Work out the finished part from the listing and answer in its coordinate system (mm). A direction names the side the tool comes from. Give positions to 0.01 mm unless a question says otherwise; leave off trailing zeros. Write each loop counter-clockwise with the first axis right and the second up, starting at its lowest first coordinate (ties: lowest second). Pieces come first, ordered by that corner, then holes.
1) Find section B-B (y = 9). Determine the outline of the cut face in (x, z).
2) Straight lines are drawn through the part: probe 1 along Y at (x, z) = (8.5, 5); probe 2 along X at (y, z) = (2.5, 2.5); probe 3 along Y at (x, z) = (51, 9.25). For each, find the intervals that lie inside material, in ascending order.
3) Given pin 1 Ø9.5 at (x, y) = (10.5, 6.5) entering from +Z; pin 2 Ø1 at (x, y) = (45, -1) entering from +Z; pin 3 Ø1.2 at (y, z) = (2.5, 5) entering from +X, each flat-ended and moving along its own axis, determine where each tip first touches the part or whether it passes through.
4) Find section C-C (z = 1.75). Determine the outline of the cut face in (x, y).
5) Find section D-D (z = 12.5). Determine the outline of the cut face in (x, y).
6) A tool of negligible diameter and unlimited length cuts with its end or side. For faces 4 (the face through (53.5, 6, 5)), 5 (the face through (65, 9, 5)), 6 (the face through (38, 0, 12)), from which of +Z, -Z, +X, -X, +Y, -Y can it reach the whole face along a straight path? Write none if from no direction.
7) Find section A-A (x = 49). Determine the outline of the cut face in (y, z), plus the area to 3 significant figures.
8) Determine the mould class of faces 1 (the face through (38, -5, 10)), 2 (the face through (65, -2, 20)), 3 (the face through (12, 3, 5)) for opening direction Y: pulls with the +Y half, pulls with the -Y half, needs draft (parallel to the pull), parting line crosses it, or undercut.
```python
from build123d import *

# Parameters (mm, degrees)
SKETCH1_W           = 77
SKETCH1_H           = 12
BOSS_EXTRUDE1_DEPTH = 10
SKETCH2_R           = 1.25
CUT_EXTRUDE1_DEPTH  = 12
SKETCH3_W           = 77
SKETCH3_H           = 20
BOSS_EXTRUDE2_DEPTH = 5
SKETCH4_W           = 30
SKETCH4_H           = 6
CUT_EXTRUDE2_DEPTH  = 10
SKETCH5_W           = 30
SKETCH5_H           = 2.5
CUT_EXTRUDE3_DEPTH  = 5


with BuildPart() as part:
    # Sketch1 → Boss-Extrude1 (new body)
    with BuildSketch(Plane.XY):
        with Locations((38.5, 6)):
            Rectangle(SKETCH1_W, SKETCH1_H)
    extrude(amount=BOSS_EXTRUDE1_DEPTH)

    # Sketch2 → Cut-Extrude1 (cut)
    with BuildSketch(Plane(origin=(77, 0, 0), x_dir=(0, 0, -1), z_dir=(1, 0, 0))):
        with Locations((-5, 3)):
            Circle(SKETCH2_R)
        with Locations((-5, 9)):
            Circle(SKETCH2_R)
    cut_extrude1 = extrude(amount=-CUT_EXTRUDE1_DEPTH, mode=Mode.SUBTRACT)

    # Mirror1: Cut-Extrude1 across plane
    add(cut_extrude1.mirror(Plane.ZY.offset(-38.5)), mode=Mode.SUBTRACT)

    # Sketch3 → Boss-Extrude2 (add)
    with BuildSketch(Plane(origin=(0, 12, 0), x_dir=(1, 0, 0), z_dir=(0, 1, 0))):
        with Locations((38.5, -10)):
            Rectangle(SKETCH3_W, SKETCH3_H)
    boss_extrude2 = extrude(amount=BOSS_EXTRUDE2_DEPTH)

    # Mirror2: Boss-Extrude2 across plane
    add(boss_extrude2.mirror(Plane(origin=(0, 6, 0), x_dir=(0, 0, 1), z_dir=(0, -1, 0))))

    # Sketch4 → Cut-Extrude2 (cut)
    with BuildSketch(Plane(origin=(0, 0, 0), x_dir=(-1, 0, 0), z_dir=(0, 0, -1))):
        with Locations((-38.5, 9)):
            Rectangle(SKETCH4_W, SKETCH4_H)
        with Locations((-38.5, 3)):
            Rectangle(SKETCH4_W, SKETCH4_H)
    extrude(amount=-CUT_EXTRUDE2_DEPTH, mode=Mode.SUBTRACT)

    # Sketch5 → Cut-Extrude3 (cut)
    with BuildSketch(Plane.XY.offset(20)):
        with Locations((38.5, -1.25)):
            Rectangle(SKETCH5_W, SKETCH5_H)
        with Locations((38.5, -3.75)):
            Rectangle(SKETCH5_W, SKETCH5_H)
    extrude(amount=-CUT_EXTRUDE3_DEPTH, mode=Mode.SUBTRACT)


solid = part.part
```
Results:
1. outline: (0, 0) - (23.5, 0) - (23.5, 10) - (0, 10) - (0, 6.25) - (12, 6.25) - (12, 3.75) - (0, 3.75) - close; (53.5, 0) - (77, 0) - (77, 3.75) - (65, 3.75) - (65, 6.25) - (77, 6.25) - (77, 10) - (53.5, 10) - close
2. probe 1: y = -5 to 1.75, 4.25 to 7.75, 10.25 to 17
2. probe 2: x = 0 to 23.5, 53.5 to 77
2. probe 3: y = -5 to 0, 12 to 17
3. pin 1: stops at z = 10
3. pin 2: stops at z = 15
3. pin 3: stops at x = 65
4. outline: (0, -5) - (77, -5) - (77, 17) - (0, 17) - close; hole (23.5, 0) - (53.5, 0) - (53.5, 12) - (23.5, 12) - close
5. outline: (0, -5) - (77, -5) - (77, 0) - (0, 0) - close; (0, 12) - (77, 12) - (77, 17) - (0, 17) - close
6. face 4: +Z, -Z
6. face 5: +X
6. face 6: +Z
7. outline: (-5, 0) - (0, 0) - (0, 15) - (-5, 15) - close; (12, 0) - (17, 0) - (17, 20) - (12, 20) - close
7. area: 175 mm2
8. face 1: pulls with the -Y half
8. face 2: needs draft
8. face 3: undercut
